```python
from build123d import *

# Parameters (mm, degrees)
SKETCH1_R           = 1.5
BOSS_EXTRUDE1_DEPTH = 5.9944


with BuildPart() as part:
    # Sketch1 → Boss-Extrude1 (new body)
    with BuildSketch(Plane.XY):
        with BuildLine():
            Line((-12.7, -25.303097847), (-12.7, -30))
            Line((-12.7, -30), (-12.7, -35.9944))
            Line((-12.7, -35.9944), (-6.35, -35.9944))
            Line((-6.35, -35.9944), (-6.35, -30))
            Line((-6.35, -30), (6.35, -30))
            Line((6.35, -30), (6.35, -35.9944))
            Line((6.35, -35.9944), (12.7, -35.9944))
            Line((12.7, -35.9944), (12.7, -30))
            Line((12.7, -30), (12.7, -25.303097847))
            ThreePointArc((12.7, -25.303097847), (12.649253454, -24.797907547), (12.499041543, -24.312903594))
            Line((12.499041543, -24.312903594), (3.694269669, -3.514229875))
            ThreePointArc((3.694269669, -3.514229875), (3.493316902, -2.529412233), (3.690098601, -1.543752674))
            ThreePointArc((3.690098601, -1.543752674), (0, 4), (-3.690098601, -1.543752674))
            ThreePointArc((-3.690098601, -1.543752674), (-3.493316902, -2.529412233), (-3.694269669, -3.514229875))
            Line((-3.694269669, -3.514229875), (-12.499041543, -24.312903594))
            ThreePointArc((-12.499041543, -24.312903594), (-12.649253454, -24.797907547), (-12.7, -25.303097847))
        make_face()
        with BuildLine():
            ThreePointArc((-2.54, -23.4976), (-2.688789755, -23.856810245), (-3.048, -24.0056))
            Line((-3.048, -24.0056), (-7.189093556, -24.0056))
            ThreePointArc((-7.189093556, -24.0056), (-7.612571853, -23.778188902), (-7.656901865, -23.299561149))
            Line((-7.656901865, -23.299561149), (-3.515808309, -13.517450387))
            ThreePointArc((-3.515808309, -13.517450387), (-2.94696194, -13.217638546), (-2.54, -13.715489237))
            Line((-2.54, -13.715489237), (-2.54, -23.4976))
        make_face(mode=Mode.SUBTRACT)
        with BuildLine():
            ThreePointArc((7.656901865, -23.299561149), (7.612571853, -23.778188902), (7.189093556, -24.0056))
            Line((7.189093556, -24.0056), (3.048, -24.0056))
            ThreePointArc((3.048, -24.0056), (2.688789755, -23.856810245), (2.54, -23.4976))
            Line((2.54, -23.4976), (2.54, -13.715489237))
            ThreePointArc((2.54, -13.715489237), (2.94696194, -13.217638546), (3.515808309, -13.517450387))
            Line((3.515808309, -13.517450387), (7.656901865, -23.299561149))
        make_face(mode=Mode.SUBTRACT)
        Circle(SKETCH1_R, mode=Mode.SUBTRACT)
    extrude(amount=BOSS_EXTRUDE1_DEPTH)


solid = part.part
```
The model under review builds one solid part; all positions refer to its coordinate system, in mm. A direction names the side the tool comes from. Give positions to 0.01 mm unless a question says otherwise; leave off trailing zeros. Loops run counter-clockwise (first coordinate to the right, second up) from the corner with the lowest first, then second, coordinate; pieces in that order, holes last. Notation, with made-up numbers: (76, 86) - (120, 86) arc R18 ccw to (120, 90) - close; hole circle Ø5 at (30.5, 69.25). An arc over 180 degrees is marked (long way). Answer as a JSON object with one key per item and string values.
Q1. Insertion check: pin 1 (1.5 mm diameter, centred on x = -2, y = -31.5, fed in from -Z); pin 2 (2 mm diameter, centred on y = -19, z = 4, fed in from +X); pin 3 (1.2 mm diameter, centred on x = 5.5, z = 3.5, fed in from +Y). Each pin has a flat end and moves straight along its axis. Give the tip position at first contact, or say it passes through.
Worked out:
{"pin 1": "passes through", "pin 2": "stops at x = 10.67", "pin 3": "stops at y = -6.36"}
Q2. Add section B-B on x = 0. State the section outline as (y, z) points, plus the area to 3 significant figures.
Worked out:
{"outline": "(-30, 0) - (-1.5, 0) - (-1.5, 5.99) - (-30, 5.99) - close; (1.5, 0) - (4, 0) - (4, 5.99) - (1.5, 5.99) - close", "area": "186 mm^2"}
Q3. Add section C-C on y = -22. State the section outline as (x, z) points.
Worked out:
{"outline": "(-11.52, 0) - (-7.11, 0) - (-7.11, 5.99) - (-11.52, 5.99) - close; (-2.54, 0) - (2.54, 0) - (2.54, 5.99) - (-2.54, 5.99) - close; (7.11, 0) - (11.52, 0) - (11.52, 5.99) - (7.11, 5.99) - close"}
Q4. To check wall thickness, follow line 1 along X through (y, z) = (-14.5, 0.7); line 2 along X through (y, z) = (-32.5, 1.6); line 3 along X through (y, z) = (-14, 1). State the ranges of each line that lie inside material, in increasing order.
Worked out:
{"line 1": "x = -8.34 to -3.93, -2.54 to 2.54, 3.93 to 8.34", "line 2": "x = -12.7 to -6.35, 6.35 to 12.7", "line 3": "x = -8.13 to -3.72, -2.54 to 2.54, 3.72 to 8.13"}
Q5. Mouldability with a two-part tool opening along Y and no side actions: class faces 1 (the flat face through (-5, -24.006, 3)), 2 (the flat face through (-6.35, -33, 3)), 3 (the cylindrical face through (-1.5, 0.07, 2.96)), 4 (the flat face through (9, -35.994, 3)) as +Y half, -Y half, draft (parallel to the pull), parting line (faces both ways), or undercut.
Worked out:
{"face 1": "undercut", "face 2": "draft", "face 3": "undercut", "face 4": "-Y half"}
Q6. For faces 5 (the flat face through (0, -30, 3)), 6 (the flat face through (2.54, -19, 3)), 7 (the flat face through (12.7, -31, 3)), list the 3-axis set-ups (+Z, -Z, +X, -X, +Y, -Y) from which the entire face can be reached by the end or side of a thin tool; tool diameter is ignored.
Worked out:
{"face 5": "+Z, -Z, -Y", "face 6": "+Z, -Z", "face 7": "+Z, -Z, +X, +Y, -Y"}
Q7. Add section A-A on y = 0. State the section outline as (x, z) points, plus the area to 3 significant figures.
Worked out:
{"outline": "(-4, 0) - (-1.5, 0) - (-1.5, 5.99) - (-4, 5.99) - close; (1.5, 0) - (4, 0) - (4, 5.99) - (1.5, 5.99) - close", "area": "30.0 mm^2"}
Q8. Add section D-D on z = 2.3. State the section outline as (x, y) points, plus the area to 3 significant figures.
Worked out:
{"outline": "(-12.7, -35.99) - (-6.35, -35.99) - (-6.35, -30) - (6.35, -30) - (6.35, -35.99) - (12.7, -35.99) - (12.7, -25.3) arc R2.54 ccw to (12.5, -24.31) - (3.69, -3.51) arc R2.54 cw to (3.69, -1.54) arc R4 ccw (long way) to (-3.69, -1.54) arc R2.54 cw to (-3.69, -3.51) - (-12.5, -24.31) arc R2.54 ccw to (-12.7, -25.3) - close; hole (-7.66, -23.3) arc R0.51 ccw to (-7.19, -24.01) - (-3.05, -24.01) arc R0.51 ccw to (-2.54, -23.5) - (-2.54, -13.72) arc R0.51 ccw to (-3.52, -13.52) - close; hole circle Ø3 at (0, 0); hole (2.54, -23.5) arc R0.51 ccw to (3.05, -24.01) - (7.19, -24.01) arc R0.51 ccw to (7.66, -23.3) - (3.52, -13.52) arc R0.51 ccw to (2.54, -13.72) - close", "area": "534 mm^2"}
